For this review, take the finished solid that the model builds, in its own axes (mm). Give positions to 0.01 mm unless a question says otherwise; leave off trailing zeros. Loops run counter-clockwise (first coordinate to the right, second up) from the corner with the lowest first, then second, coordinate; pieces in that order, holes last.
```python
from build123d import *

# Parameters (mm, degrees)
SKETCH1_R           = 19.05
SKETCH1_R_2         = 5
BOSS_EXTRUDE1_DEPTH = 9.525
CUT_EXTRUDE1_DEPTH  = 20.05


with BuildPart() as part:
    # Sketch1 → Boss-Extrude1 (new body, symmetric)
    with BuildSketch(Plane.XY):
        Circle(SKETCH1_R)
        Circle(SKETCH1_R_2, mode=Mode.SUBTRACT)
    extrude(amount=BOSS_EXTRUDE1_DEPTH, both=True)

    # Sketch2 → Cut-Extrude1 (cut, through all)
    with BuildSketch(Plane(origin=(0, 0, -9.525), x_dir=(-1, 0, 0), z_dir=(0, 0, -1))):
        with BuildLine():
            ThreePointArc((-2.382933771, -7.353538376), (-3.492043555, -6.04839686), (-5.176884156, -5.740450369))
            ThreePointArc((-5.176884156, -5.740450369), (-7.794228634, -4.5), (-7.559817926, -1.613088007))
            ThreePointArc((-7.559817926, -1.613088007), (-6.984087111, 0), (-7.559817926, 1.613088007))
            ThreePointArc((-7.559817926, 1.613088007), (-7.794228634, 4.5), (-5.176884156, 5.740450369))
            ThreePointArc((-5.176884156, 5.740450369), (-3.492043555, 6.04839686), (-2.382933771, 7.353538376))
            ThreePointArc((-2.382933771, 7.353538376), (0, 9), (2.382933771, 7.353538376))
            ThreePointArc((2.382933771, 7.353538376), (3.492043555, 6.04839686), (5.176884156, 5.740450369))
            ThreePointArc((5.176884156, 5.740450369), (7.794228634, 4.5), (7.559817926, 1.613088007))
            ThreePointArc((7.559817926, 1.613088007), (6.984087111, 0), (7.559817926, -1.613088007))
            ThreePointArc((7.559817926, -1.613088007), (7.794228634, -4.5), (5.176884156, -5.740450369))
            ThreePointArc((5.176884156, -5.740450369), (3.492043555, -6.04839686), (2.382933771, -7.353538376))
            ThreePointArc((2.382933771, -7.353538376), (0, -9), (-2.382933771, -7.353538376))
        make_face()
    extrude(amount=-CUT_EXTRUDE1_DEPTH, mode=Mode.SUBTRACT)


solid = part.part
```
Q1. For probe 1 along Y at (x, z) = (-4.5, -1.5); probe 2 along Y at (x, z) = (-5, -0.75); probe 3 along X at (y, z) = (6.5, 6), list the stretches that pass through material, from the lowest coordinate up.
Answers:
probe 1: y = -18.51 to -5.72, 5.72 to 18.51
probe 2: y = -18.38 to -5.72, 5.72 to 18.38
probe 3: x = -17.91 to -2.92, 2.92 to 17.91
Q2. Consider section D-D on x = -11. Give the boundary of the cut face in (y, z) (3 decimals), plus the area to 3 significant figures.
Answers:
outline: (-15.553, -9.525) - (15.553, -9.525) - (15.553, 9.525) - (-15.553, 9.525) - close
area: 593 mm2
Q3. Consider section C-C on z = 6.5. Give the boundary of the cut face in (x, y).
Answers:
outline: circle Ø38.1 at (0, 0); hole (-7.56, -1.61) arc R2.55 ccw to (-5.18, -5.74) arc R2.55 cw to (-2.38, -7.35) arc R2.55 ccw to (2.38, -7.35) arc R2.55 cw to (5.18, -5.74) arc R2.55 ccw to (7.56, -1.61) arc R2.55 cw to (7.56, 1.61) arc R2.55 ccw to (5.18, 5.74) arc R2.55 cw to (2.38, 7.35) arc R2.55 ccw to (-2.38, 7.35) arc R2.55 cw to (-5.18, 5.74) arc R2.55 ccw to (-7.56, 1.61) arc R2.55 cw to start
Q4. For pin 1 Ø10 at (y, z) = (-10, -5.5) entering from -X; pin 2 Ø5 at (y, z) = (13.5, 2) entering from -X, all flat-tipped, find the tip position at first contact; note any pin that passes through.
Answers:
pin 1: stops at x = -18.38
pin 2: stops at x = -15.55
Q5. Consider section A-A on x = 0. Give the boundary of the cut face in (y, z) (3 decimals).
Answers:
outline: (-19.05, -9.525) - (-9, -9.525) - (-9, 9.525) - (-19.05, 9.525) - close; (9, -9.525) - (19.05, -9.525) - (19.05, 9.525) - (9, 9.525) - close
Q6. Consider section B-B on y = 0. Give the boundary of the cut face in (x, z) (3 decimals).
Answers:
outline: (-19.05, -9.525) - (-6.984, -9.525) - (-6.984, 9.525) - (-19.05, 9.525) - close; (6.984, -9.525) - (19.05, -9.525) - (19.05, 9.525) - (6.984, 9.525) - close
